CAD build for the part. Positions are in the model's coordinates, mm. A direction names the side the tool comes from. Give positions to 0.01 mm unless a question says otherwise; leave off trailing zeros.
Item 1: Band-saw the part on A-A on x = 50.8. Count the separate pieces of the cut face and the enclosed holes in it, plus the area to 3 significant figures.
Item 2: Which spindle directions (+Z, -Z, +X, -X, +Y, -Y) get a long thin tool onto all of the face, cutting with end or side? Do faces 1 (the flat face through (81.28, 5, 2)), 2 (the cylindrical face through (51.679, 92.036, 2.447)). Say none if no direction does.
Item 3: Two-plate mould, pull along Y, no slides. Class faces 3 (the flat face through (99, 22.352, 2)), 4 (the flat face through (101.6, 11, 2)), 5 (the flat face through (91, 0, 2)): released by +Y, released by -Y, zero draft, split by the parting line, or undercut.
Item 4: Flat gauge pins, fed straight in: P1, Ø1.5, axis at x = 39, z = 3, coming from the -Y side; P2, Ø1, axis at y = 33.5, z = 1, coming from the -X side. Where does each tip first touch, or does it go through?
Item 5: Wall check: L1, parallel to X at y = 6.5, z = 4.55; L2, parallel to X at y = 67, z = 0.6; L3, parallel to X at y = 82.5, z = 2.7. Give the ranges that are in metal, low to high.
```python
from build123d import *

# Parameters (mm, degrees)
BOSS_EXTRUDE1_DEPTH = 4.826
SKETCH2_R           = 1.905
CUT_EXTRUDE1_DEPTH  = 151.366498303
SKETCH3_W           = 4.826
SKETCH3_H           = 12.7
CUT_EXTRUDE2_DEPTH  = 151.366498303


with BuildPart() as part:
    # Sketch1 → Boss-Extrude1 (new body)
    with BuildSketch(Plane.XY):
        Polygon((0, 110.744), (0, 0), (20.32, 0), (20.32, 9.652), (40.64, 9.652), (40.64, 0), (60.96, 0), (60.96, 9.652), (81.28, 9.652), (81.28, 0), (101.6, 0), (101.6, 110.744), (81.28, 110.744), (81.28, 101.092), (60.96, 101.092), (60.96, 110.744), (40.64, 110.744), (40.64, 101.092), (20.32, 101.092), (20.32, 110.744), align=None)
    extrude(amount=BOSS_EXTRUDE1_DEPTH)

    # Sketch2 → Cut-Extrude1 (cut, through all)
    with BuildSketch(Plane.XY.offset(4.826)):
        with Locations((50.8, 68.326)):
            Circle(SKETCH2_R)
        with Locations((63.5, 68.326)):
            Circle(SKETCH2_R)
        with Locations((76.2, 68.326)):
            Circle(SKETCH2_R)
        with Locations((63.5, 81.026)):
            Circle(SKETCH2_R)
        with Locations((76.2, 81.026)):
            Circle(SKETCH2_R)
        with Locations((63.5, 93.726)):
            Circle(SKETCH2_R)
        with Locations((76.2, 93.726)):
            Circle(SKETCH2_R)
        with Locations((38.1, 68.326)):
            Circle(SKETCH2_R)
        with Locations((25.4, 68.326)):
            Circle(SKETCH2_R)
        with Locations((38.1, 81.026)):
            Circle(SKETCH2_R)
        with Locations((25.4, 81.026)):
            Circle(SKETCH2_R)
        with Locations((38.1, 93.726)):
            Circle(SKETCH2_R)
        with Locations((25.4, 93.726)):
            Circle(SKETCH2_R)
        with Locations((50.8, 81.026)):
            Circle(SKETCH2_R)
        with Locations((50.8, 93.726)):
            Circle(SKETCH2_R)
        with Locations((63.5, 55.626)):
            Circle(SKETCH2_R)
        with Locations((76.2, 55.626)):
            Circle(SKETCH2_R)
        with Locations((63.5, 42.926)):
            Circle(SKETCH2_R)
        with Locations((76.2, 42.926)):
            Circle(SKETCH2_R)
        with Locations((63.5, 30.226)):
            Circle(SKETCH2_R)
        with Locations((76.2, 30.226)):
            Circle(SKETCH2_R)
        with Locations((63.5, 17.526)):
            Circle(SKETCH2_R)
        with Locations((76.2, 17.526)):
            Circle(SKETCH2_R)
        with Locations((38.1, 55.626)):
            Circle(SKETCH2_R)
        with Locations((25.4, 55.626)):
            Circle(SKETCH2_R)
        with Locations((38.1, 42.926)):
            Circle(SKETCH2_R)
        with Locations((25.4, 42.926)):
            Circle(SKETCH2_R)
        with Locations((38.1, 30.226)):
            Circle(SKETCH2_R)
        with Locations((25.4, 30.226)):
            Circle(SKETCH2_R)
        with Locations((38.1, 17.526)):
            Circle(SKETCH2_R)
        with Locations((25.4, 17.526)):
            Circle(SKETCH2_R)
        with Locations((50.8, 55.626)):
            Circle(SKETCH2_R)
        with Locations((50.8, 42.926)):
            Circle(SKETCH2_R)
        with Locations((50.8, 30.226)):
            Circle(SKETCH2_R)
        with Locations((50.8, 17.526)):
            Circle(SKETCH2_R)
    extrude(amount=-CUT_EXTRUDE1_DEPTH, mode=Mode.SUBTRACT)

    # Sketch3 → Cut-Extrude2 (cut, through all)
    with BuildSketch(Plane.XY.offset(4.826)):
        with Locations((2.413, 28.702)):
            Rectangle(SKETCH3_W, SKETCH3_H)
        with Locations((99.187, 28.702)):
            Rectangle(SKETCH3_W, SKETCH3_H)
    extrude(amount=-CUT_EXTRUDE2_DEPTH, mode=Mode.SUBTRACT)


solid = part.part
```
The answers:
1. separate pieces: 8
1. enclosed holes: 0
1. area: 406 mm2
2. face 1: +Z, -Z, -Y
2. face 2: +Z, -Z
3. face 3: undercut
3. face 4: zero draft
3. face 5: released by -Y
4. P1: stops at y = 9.65
4. P2: stops at x = 4.83
5. L1: x = 0 to 20.32, 40.64 to 60.96, 81.28 to 101.6
5. L2: x = 0 to 24.03, 26.77 to 36.73, 39.47 to 49.43, 52.17 to 62.13, 64.87 to 74.83, 77.57 to 101.6
5. L3: x = 0 to 24.19, 26.61 to 36.89, 39.31 to 49.59, 52.01 to 62.29, 64.71 to 74.99, 77.41 to 101.6
